Design review of the part built by this model. Coordinates are the model's own, in mm. Face numbers are marked on the shaded views. A direction names the side the tool comes from. Coordinates: 2 decimals unless noted, no trailing zeros. Write each loop counter-clockwise with the first axis right and the second up, starting at its lowest first coordinate (ties: lowest second). Pieces come first, ordered by that corner, then holes. Notation, with made-up numbers: (81, 32.25) -> (97, 32.25) arc R17 ccw to (97, 64.25) -> close; hole circle Ø4 at (88.25, 37.25). An arc over 180 degrees is marked (long way). Answer in a Markdown table with one row per item. Add a question column.
Item 1: Clearance check with flat-ended pins moving along their axes: P1, Ø1, axis at y = 0.5, z = 11, coming from the +X side; P2, Ø2, axis at x = 94, z = 12.5, coming from the +Y side; P3, Ø4, axis at x = 0, y = 0, coming from the +Z side. State where each tip first meets the part, or that it passes through.
Item 2: For the marked faces 1, 2 and 3, list the 3-axis set-ups (+Z, -Z, +X, -X, +Y, -Y) from which the entire face can be reached by the end or side of a thin tool; tool diameter is ignored.
Item 3: Take a section at A-A, the plane y = 0. Give the number of separate pieces and of enclosed holes in the cut face, and give its area (3 significant figures).
Item 4: Take a section at D-D, the plane x = 42. Write out the cut boundary in (y, z).
Item 5: To check wall thickness, follow line 1 (Y direction, x = 150, z = 9.3); line 2 (Y direction, x = 0, z = 20.25); line 3 (Z direction, x = 34, y = -6). State the ranges of each line that lie inside material, in increasing order.
Item 6: Take a section at C-C, the plane x = 158. Write out the cut boundary in (y, z).
Item 7: Take a section at B-B, the plane z = 6.25. Write out the cut boundary in (x, y).
from build123d import *
from OCP.BRepFilletAPI import BRepFilletAPI_MakeChamfer

# Parameters (mm, degrees)
EXTRUDE_1_DEPTH     = 22
SKETCH_2_R          = 10.5
CUT_EXTRUDE_1_DEPTH = 4.2
CUT_EXTRUDE_START   = -9.4
CUT_EXTRUDE_6_DEPTH = 9.4
CUT_EXTRUDE_7_DEPTH = 9.4
SKETCH_4_R          = 10.5
CUT_EXTRUDE_2_DEPTH = 4.2
SKETCH_8_R          = 1.6
CUT_EXTRUDE_5_DEPTH = 173.095438638
CHAMFER_1_SIZE      = 4.7
CHAMFER_1_SIZE2     = 26.655024552
CHAMFER_2_SIZE2     = 26.655024552
CHAMFER_2_SIZE      = 4.7
CHAMFER_3_SIZE2     = 4.7
CHAMFER_3_SIZE      = 26.655024552
FILLET_4_R          = 10


with BuildPart() as part:
    # 草图1 → 凸台-拉伸1 (new body)
    with BuildSketch(Plane.XY):
        with BuildLine():
            Line((0, 16), (150, 20))
            ThreePointArc((150, 20), (170, 0), (150, -20))
            Line((150, -20), (0, -16))
            ThreePointArc((0, -16), (-16, 0), (0, 16))
        make_face()
    extrude(amount=EXTRUDE_1_DEPTH)

    # 草图2 → 切除-拉伸1 (cut)
    with BuildSketch(Plane.XY.offset(22)):
        Circle(SKETCH_2_R)
    extrude(amount=-CUT_EXTRUDE_1_DEPTH, mode=Mode.SUBTRACT)

    # 草图9 → 切除-拉伸6 (cut)
    with BuildSketch(Plane.XY.offset(22).offset(CUT_EXTRUDE_START)):
        with BuildLine():
            Line((75, 18), (75, -18))
            Line((75, -18), (150, -20))
            ThreePointArc((150, -20), (170, 0), (150, 20))
            Line((150, 20), (75, 18))
        make_face()
    extrude(amount=CUT_EXTRUDE_6_DEPTH, mode=Mode.SUBTRACT)

    # 草图10 → 切除-拉伸7 (cut)
    with BuildSketch(Plane(origin=(0, 0, 0), x_dir=(-1, 0, 0), z_dir=(0, 0, -1))):
        with BuildLine():
            Line((-75, 18), (-75, -18))
            Line((-75, -18), (0, -16))
            ThreePointArc((0, -16), (16, 0), (0, 16))
            Line((0, 16), (-75, 18))
        make_face()
    extrude(amount=-CUT_EXTRUDE_7_DEPTH, mode=Mode.SUBTRACT)

    # 草图4 → 切除-拉伸2 (cut)
    with BuildSketch(Plane(origin=(0, 0, 12.6), x_dir=(-1, 0, 0), z_dir=(0, 0, -1))):
        with Locations((-150, 0)):
            Circle(SKETCH_4_R)
    extrude(amount=CUT_EXTRUDE_2_DEPTH, mode=Mode.SUBTRACT)

    # 草图8 → 切除-拉伸5 (cut, through all)
    with BuildSketch(Plane.XY.offset(17.8)):
        Circle(SKETCH_8_R)
        with Locations((150, 0)):
            Circle(SKETCH_8_R)
    extrude(amount=-CUT_EXTRUDE_5_DEPTH, mode=Mode.SUBTRACT)

    # 倒角1: one chamfer whose edges measure the first distance from different faces: ONE call of the kernel's chamfer builder (chamfer() names one face for all edges)
    chamfer_1_edges_1 = [part.edges().sort_by_distance(p)[0] for p in [
        (75, 0, 12.6),
    ]]
    chamfer_1_side_1 = [part.faces().sort_by_distance(p)[0] for p in [
        (75, 0, 17.3),
    ]]
    chamfer_1_edges_2 = [part.edges().sort_by_distance(p)[0] for p in [
        (75, 0, 9.4),
    ]]
    chamfer_1_side_2 = [part.faces().sort_by_distance(p)[0] for p in [
        (75, 0, 4.7),
    ]]
    chamfer_1 = BRepFilletAPI_MakeChamfer(part.part.solid().wrapped)
    for e in chamfer_1_edges_1:
        chamfer_1.Add(CHAMFER_1_SIZE, CHAMFER_1_SIZE2, e.wrapped, chamfer_1_side_1[0].wrapped)  # the first distance lies on this face
    for e in chamfer_1_edges_2:
        chamfer_1.Add(CHAMFER_1_SIZE, CHAMFER_1_SIZE2, e.wrapped, chamfer_1_side_2[0].wrapped)  # the first distance lies on this face
    add(Compound.cast(chamfer_1.Shape()), mode=Mode.REPLACE)

    # 倒角2
    chamfer_2_edges = [part.edges().sort_by_distance(p)[0] for p in [
        (75, 0, 22),
    ]]
    chamfer_2_side = [part.faces().sort_by_distance(p)[0] for p in [
        (75, 0, 21.906),
    ]]
    chamfer(chamfer_2_edges, length=CHAMFER_2_SIZE - 0.0001, length2=CHAMFER_2_SIZE2 - 0.0001, reference=chamfer_2_side[0])  # a hair under: the kernel refuses the full size

    # 倒角3
    chamfer_3_edges = [part.edges().sort_by_distance(p)[0] for p in [
        (75, 0, 0),
    ]]
    chamfer_3_side = [part.faces().sort_by_distance(p)[0] for p in [
        (75.094, 0, 0),
    ]]
    chamfer(chamfer_3_edges, length=CHAMFER_3_SIZE - 0.0001, length2=CHAMFER_3_SIZE2 - 0.0001, reference=chamfer_3_side[0])  # a hair under: the kernel refuses the full size

    # 圆角4
    fillet_4_edges = [part.edges().sort_by_distance(p)[0] for p in [
        (101.655024552, 0, 12.6),
        (48.344975448, 0, 9.4),
        (48.345075448, 0, 22),
        (101.654924552, 0, 0),
    ]]
    fillet(fillet_4_edges, radius=FILLET_4_R)


solid = part.part
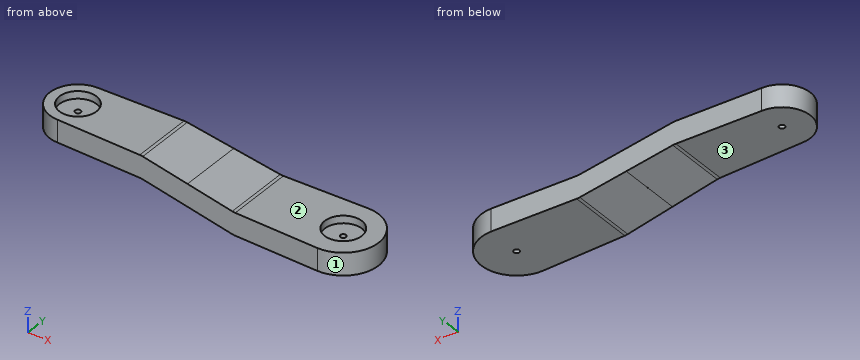
Answers:
| question | item | result |
|---|---|---|
| 1 | P1 | stops at x = 170 |
| 1 | P2 | stops at y = 18.53 |
| 1 | P3 | stops at z = 17.8 |
| 2 | face 1 | +Z, -Z, +X |
| 2 | face 2 | +Z, +X, +Y, -Y |
| 2 | face 3 | -Z, -X, +Y, -Y |
| 3 | separate pieces | 3 |
| 3 | enclosed holes | 0 |
| 3 | area | 2,110 mm^2 |
| 4 | outline | (-17.12, 9.4) -> (17.12, 9.4) -> (17.12, 22) -> (-17.12, 22) -> close |
| 5 | line 1 | y = -20 to -10.5, 10.5 to 20 |
| 5 | line 2 | y = -16 to -10.5, 10.5 to 16 |
| 5 | line 3 | z = 9.4 to 22 |
| 6 | outline | (-18.33, 0) -> (18.33, 0) -> (18.33, 12.6) -> (6.8, 12.6) -> (6.8, 8.4) -> (-6.8, 8.4) -> (-6.8, 12.6) -> (-18.33, 12.6) -> close |
| 7 | outline | (66.21, -17.77) -> (150, -20) arc R20 ccw to (150, 20) -> (66.21, 17.77) -> close; hole circle Ø3.2 at (150, 0) |
